Part model, mm, in its own coordinate system. A direction names the side the tool comes from. Give positions to 0.01 mm unless a question says otherwise; leave off trailing zeros. Write each loop counter-clockwise with the first axis right and the second up, starting at its lowest first coordinate (ties: lowest second). Pieces come first, ordered by that corner, then holes. Notation, with made-up numbers: (30.5, 3.25) - (84.5, 3.25) arc R23 ccw to (84.5, 11.25) - close; hole circle Ø2 at (-16, 60). An arc over 180 degrees is marked (long way). Answer in a Markdown table with one row per item. Add a question column.
1. Band-saw the part on C-C on x = 104. Write the cut outline in (y, z), plus the area to 3 significant figures.
2. Band-saw the part on D-D on z = 2.85. State how many separate pieces and enclosed holes the cut face has, plus the area to 3 significant figures.
3. Probe line 1 along X through (y, z) = (10, 1.8); line 2 along Y through (x, z) = (130, 3.35); line 3 along X through (y, z) = (114.5, 4). List the from-to ranges inside material, lowest first.
4. Band-saw the part on A-A on y = 77.5. Write the cut outline in (x, z), plus the area to 3 significant figures.
5. Pull direction X, two halves, no side cores. Call faces 3 (the cylindrical face through (28.22, 115.41, 2.46)), 4 (the flat face through (0, 51, 2)), 5 (the flat face through (101, 160, 2)), 6 (the flat face through (140, 79, 2)): released by +X, released by -X, zero draft, split by the parting line, or undercut.
6. Which spindle directions (+Z, -Z, +X, -X, +Y, -Y) get a long thin tool onto all of the face, cutting with end or side? Do faces 1 (the flat face through (69, 81, 0)), 2 (the cylindrical face through (57.74, 157.64, 2.46)). Say none if no direction does.
7. Band-saw the part on B-B on y = 115. Write the cut outline in (x, z) (3 decimals).
8. Drop flat-ended pins along their axis: pin 1 Ø3 at (y, z) = (129, 3.5) entering from -X; pin 2 Ø6 at (x, y) = (41, 77.5) entering from +Z. Give the stop position or say it passes through.
```python
from build123d import *

# Parameters (mm, degrees)
MODEL_R             = 3
MODEL_R_2           = 2.25
MODEL_R_3           = 1.25
MODEL_R_4           = 12.5
MODEL_R_5           = 3.25
MODEL_R_6           = 14.225
BOSS_EXTRUDE1_DEPTH = 5


with BuildPart() as part:
    # Model → Boss-Extrude1 (new body)
    with BuildSketch(Plane.XY):
        with BuildLine():
            Line((28.011750385, 160), (2, 160))
            ThreePointArc((2, 160), (0.585786438, 159.414213562), (0, 158))
            Line((0, 158), (0, 131.988249615))
            ThreePointArc((0, 131.988249615), (2.421581013, 127.704354714), (7.340702211, 127.569979234))
            ThreePointArc((7.340702211, 127.569979234), (28.225, 115), (7.340702211, 102.430020766))
            ThreePointArc((7.340702211, 102.430020766), (2.421581013, 102.295645286), (0, 98.011750385))
            Line((0, 98.011750385), (0, 2))
            ThreePointArc((0, 2), (0.585786438, 0.585786438), (2, 0))
            Line((2, 0), (138, 0))
            ThreePointArc((138, 0), (139.414213562, 0.585786438), (140, 2))
            Line((140, 2), (140, 158))
            ThreePointArc((140, 158), (139.414213562, 159.414213562), (138, 160))
            Line((138, 160), (61.988249616, 160))
            ThreePointArc((61.988249616, 160), (57.704354714, 157.578418987), (57.569979234, 152.659297789))
            ThreePointArc((57.569979234, 152.659297789), (45, 131.775), (32.430020766, 152.659297789))
            ThreePointArc((32.430020766, 152.659297789), (32.295645286, 157.578418987), (28.011750385, 160))
        make_face()
        with Locations((26, 91.5)):
            Circle(MODEL_R, mode=Mode.SUBTRACT)
        with Locations((55, 77.5)):
            Circle(MODEL_R_2, mode=Mode.SUBTRACT)
        with Locations((55, 60)):
            Circle(MODEL_R_3, mode=Mode.SUBTRACT)
        with Locations((109, 77.5)):
            Circle(MODEL_R_4, mode=Mode.SUBTRACT)
        with Locations((55, 95)):
            Circle(MODEL_R_3, mode=Mode.SUBTRACT)
        with Locations((26, 63.5)):
            Circle(MODEL_R, mode=Mode.SUBTRACT)
        with Locations((41, 77.5)):
            Circle(MODEL_R_5, mode=Mode.SUBTRACT)
        with Locations((45, 115)):
            Circle(MODEL_R_6, mode=Mode.SUBTRACT)
        with BuildLine():
            Line((5, 153), (5, 150))
            ThreePointArc((5, 150), (13.535533906, 146.464466094), (10, 155))
            Line((10, 155), (7, 155))
            ThreePointArc((7, 155), (5.585786438, 154.414213562), (5, 153))
        make_face(mode=Mode.SUBTRACT)
        with BuildLine():
            Line((7, 5), (10, 5))
            ThreePointArc((10, 5), (13.535533906, 13.535533906), (5, 10))
            Line((5, 10), (5, 7))
            ThreePointArc((5, 7), (5.585786438, 5.585786438), (7, 5))
        make_face(mode=Mode.SUBTRACT)
        with BuildLine():
            Line((135, 7), (135, 10))
            ThreePointArc((135, 10), (126.464466094, 13.535533906), (130, 5))
            Line((130, 5), (133, 5))
            ThreePointArc((133, 5), (134.414213562, 5.585786438), (135, 7))
        make_face(mode=Mode.SUBTRACT)
        with BuildLine():
            Line((133, 155), (130, 155))
            ThreePointArc((130, 155), (126.464466094, 146.464466094), (135, 150))
            Line((135, 150), (135, 153))
            ThreePointArc((135, 153), (134.414213562, 154.414213562), (133, 155))
        make_face(mode=Mode.SUBTRACT)
    extrude(amount=BOSS_EXTRUDE1_DEPTH)


solid = part.part
```
Values:
| question | item | result |
|---|---|---|
| 1 | outline | (0, 0) - (66.04, 0) - (66.04, 5) - (0, 5) - close; (88.96, 0) - (160, 0) - (160, 5) - (88.96, 5) - close |
| 1 | area | 685 mm² |
| 2 | separate pieces | 1 |
| 2 | enclosed holes | 12 |
| 2 | area | 19,400 mm² |
| 3 | line 1 | x = 0 to 5, 15 to 125, 135 to 140 |
| 3 | line 2 | y = 0 to 5, 15 to 145, 155 to 160 |
| 3 | line 3 | x = 28.22 to 30.78, 59.22 to 140 |
| 4 | outline | (0, 0) - (37.75, 0) - (37.75, 5) - (0, 5) - close; (44.25, 0) - (52.75, 0) - (52.75, 5) - (44.25, 5) - close; (57.25, 0) - (96.5, 0) - (96.5, 5) - (57.25, 5) - close; (121.5, 0) - (140, 0) - (140, 5) - (121.5, 5) - close |
| 4 | area | 520 mm² |
| 5 | face 3 | undercut |
| 5 | face 4 | released by -X |
| 5 | face 5 | zero draft |
| 5 | face 6 | released by +X |
| 6 | face 1 | -Z, +X, -X, +Y, -Y |
| 6 | face 2 | +Z, -Z |
| 7 | outline | (28.225, 0) - (30.775, 0) - (30.775, 5) - (28.225, 5) - close; (59.225, 0) - (140, 0) - (140, 5) - (59.225, 5) - close |
| 8 | pin 1 | stops at x = 0.23 |
| 8 | pin 2 | passes through |
